from build123d import *

# Parameters (mm, degrees)
F0_W     = 254
F0_H     = 203.2
F0_W_2   = 76.2
F0_H_2   = 76.2
F1_DEPTH = 25.4
F2_DEPTH = 50.8
F3_DEPTH = 762


with BuildPart() as f1:
    # F0 (on Top) → F1 (new body)
    with BuildSketch(Plane.XY):
        with Locations((127, -101.6)):
            Rectangle(F0_W, F0_H)
        Polygon((457.2, 0), (254, 0), (254, -203.2), (0, -203.2), (0, -914.4), (457.2, -914.4), (457.2, -457.2), (381, -457.2), (381, -381), (457.2, -381), align=None)
        with Locations((419.1, -419.1)):
            Rectangle(F0_W_2, F0_H_2)
    extrude(amount=-F1_DEPTH)

    # F0 (on Top) → F2 (join)
    with BuildSketch(Plane.XY):
        with Locations((127, -101.6)):
            Rectangle(F0_W, F0_H)
    extrude(amount=F2_DEPTH)

    # F0 (on Top) → F3 (join)
    with BuildSketch(Plane.XY):
        with Locations((419.1, -419.1)):
            Rectangle(F0_W_2, F0_H_2)
    extrude(amount=F3_DEPTH)


solid = f1.part
Source: CAD feature listing. Evaluate the final solid. Frame: model axes, mm. A direction names the side the tool comes from. Round coordinates to 2 decimals unless told otherwise and drop trailing zeros. Loops run counter-clockwise (first coordinate to the right, second up) from the corner with the lowest first, then second, coordinate; pieces in that order, holes last. Notation, with made-up numbers: (74, 53.5) -> (126, 53.5) arc R10 cw to (126, 62.5) -> close; hole circle Ø11 at (16, 20). An arc over 180 degrees is marked (long way). Answer as a JSON object with one key per item and string values. Group by question number.
Q1. Section query D-D (x = 289). Output: boundary loops of the cut face in (y, z), plus the area to 3 significant figures.
Q2. Ray query, line 1 (Y direction, x = 433, z = 569); line 2 (Z direction, x = 22, y = -100); line 3 (Z direction, x = 262.5, y = -454.5). Return the intervals inside material, ascending. Write a range as from..to.
Q3. Section query B-B (y = -424.5). Output: boundary loops of the cut face in (x, z).
Q4. Contact query for flat-ended pins moving along their axis: P1, Ø1.5, axis at x = 90, y = -778, coming from the +Z side; P2, Ø15, axis at y = -105.5, z = 14.5, coming from the +X side; P3, Ø23, axis at y = -432.5, z = 405.5, coming from the -X side. Output: stop coordinate, or through.
Q5. Access query for faces 1 (the flat face through (254, -103, 25)), 2 (the flat face through (419, -381, 376)), 3 (the flat face through (381, -420, 376)), 4 (the flat face through (419, -457.2, 376)). Directions: +Z, -Z, +X, -X, +Y, -Y. A direction counts if a zero-diameter tool reaches every point of the face in a straight line with its end or side. Return the directions, or none.
Q6. Section query A-A (x = 59). Output: boundary loops of the cut face in (y, z).
Q7. Section query C-C (z = 326). Output: boundary loops of the cut face in (x, y).
Completed:
{
 "1": {"outline": "(-914.4, -25.4) -> (0, -25.4) -> (0, 0) -> (-914.4, 0) -> close", "area": "23,200 mm²"},
 "2": {"line 1": "-457.2..-381", "line 2": "-25.4..50.8", "line 3": "-25.4..0"},
 "3": {"outline": "(0, -25.4) -> (457.2, -25.4) -> (457.2, 762) -> (381, 762) -> (381, 0) -> (0, 0) -> close"},
 "4": {"P1": "z = 0", "P2": "x = 254", "P3": "x = 381"},
 "5": {"face 1": "+Z, +X, +Y, -Y", "face 2": "+Z, +X, -X, +Y", "face 3": "+Z, -X, +Y, -Y", "face 4": "+Z, +X, -X, -Y"},
 "6": {"outline": "(-914.4, -25.4) -> (0, -25.4) -> (0, 50.8) -> (-203.2, 50.8) -> (-203.2, 0) -> (-914.4, 0) -> close"},
 "7": {"outline": "(381, -457.2) -> (457.2, -457.2) -> (457.2, -381) -> (381, -381) -> close"}
}
